The listing builds one solid part. Answer for the finished solid, in the listing's coordinates (mm). Coordinates: 2 decimals unless noted, no trailing zeros. Order: outer loops, then holes, each group sorted by start corner. A loop starts at its lowest first (then second) coordinate and runs counter-clockwise, first axis right, second up. Notation, with made-up numbers: (65, 63) -> (123, 63) arc R15 cw to (123, 88) -> close; hole circle Ø4 at (55.25, -11.5). An arc over 180 degrees is marked (long way). One line per question, with ' | ' between items.
Autodesk Inventor part; units mm, degrees
ref_plane "YZ Plane" through (0, 0, 0) normal (1, 0, 0) x (0, 1, 0)
ref_plane "XZ Plane" through (0, 0, 0) normal (0, 1, 0) x (-1, 0, 0)
ref_plane "XY Plane" through (0, 0, 0) normal (0, 0, 1) x (1, 0, 0)
sketch "Sketch1" plane through (0, 0, 0) normal (1, 0, 0) x (0, 1, 0)
  line L0 (15, 30) -> (-15, 30)
  line L1 (-15, 30) -> (-15, -30)
  line L2 (-15, -30) -> (15, -30)
  line L3 (15, -30) -> (15, 30)
  line L4 (15, 30) -> (-15, -30) construction
  line L5 (-15, 30) -> (15, -30) construction
  line L6 (15, 30) -> (18, 30)
  line L7 (18, 30) -> (18, 20)
  line L8 (18, 20) -> (15, 20)
  line L9 (15, 20) -> (15, 30)
  line L10 (15, -30) -> (18, -30)
  line L11 (18, -30) -> (18, -20)
  line L12 (18, -20) -> (15, -20)
  line L13 (15, -20) -> (15, -30)
  line L14 (15, 5) -> (18, 5)
  line L15 (18, 5) -> (18, -5)
  line L16 (18, -5) -> (15, -5)
  line L17 (15, -5) -> (15, 5)
  point P0 (0, 0)
  point P1 (18, 0)
  point P2 (0, 0)
  dimension "d0" = 30
  dimension "d1" = 60
  dimension "d2" = 3
  dimension "d3" = 10
  dimension "d4" = 3
  dimension "d5" = 10
  dimension "d6" = 3
  dimension "d7" = 10
extrude "Extrusion1" add sketch "Sketch1" along normal blind 3
sketch "Sketch2" plane through (0, 0, 0) normal (-1, 0, 0) x (0, 0, 1)
  line L0 (25, 10) -> (-25, 10)
  line L1 (-25, 10) -> (-25, -10)
  line L2 (-25, -10) -> (25, -10)
  line L3 (25, -10) -> (25, 10)
  line L4 (25, 10) -> (-25, -10) construction
  line L5 (-25, 10) -> (25, -10) construction
  line L6 (30, -15) -> (-30, -15)
  line L7 (-30, -15) -> (-30, 18)
  point P0 (0, 0)
  dimension "d10" = 5
  dimension "d11" = 5
extrude "Extrusion2" cut sketch "Sketch2" against normal blind 3
sketch "Sketch3" plane through (0, 0, 0) normal (-1, 0, 0) x (0, 0, 1)
  line L0 (-25, -10) -> (-25, 10)
  line L1 (-25, 10) -> (25, 10)
  line L2 (25, 10) -> (25, -10)
  line L3 (25, -10) -> (-25, -10)
  line L4 (-30, -15) -> (-30, 18)
  line L5 (30, -15) -> (-30, -15)
  line L6 (30, 18) -> (30, -15)
  line L7 (20, 18) -> (30, 18)
  line L8 (20, 15) -> (20, 18)
  line L9 (5, 15) -> (20, 15)
  line L10 (5, 18) -> (5, 15)
  line L11 (-5, 18) -> (5, 18)
  line L12 (-5, 15) -> (-5, 18)
  line L13 (-20, 15) -> (-5, 15)
  line L14 (-20, 18) -> (-20, 15)
  line L15 (-30, 18) -> (-20, 18)
  line L16 (25.5571, 8.6073) -> (-24.4429, -11.3927)
  line L17 (-24.4429, -11.3927) -> (-25.5571, -8.6073)
  line L18 (-25.5571, -8.6073) -> (24.4429, 11.3927)
  line L19 (24.4429, 11.3927) -> (25.5571, 8.6073)
  line L20 (25.5571, 8.6073) -> (-25.5571, -8.6073) construction
  line L21 (-24.4429, -11.3927) -> (24.4429, 11.3927) construction
  line L22 (-25.5571, 8.6073) -> (24.4429, -11.3927)
  line L23 (24.4429, -11.3927) -> (25.5571, -8.6073)
  line L24 (25.5571, -8.6073) -> (-24.4429, 11.3927)
  line L25 (-24.4429, 11.3927) -> (-25.5571, 8.6073)
  line L26 (-25.5571, 8.6073) -> (25.5571, -8.6073) construction
  line L27 (24.4429, -11.3927) -> (-24.4429, 11.3927) construction
  point P0 (0, 0)
  dimension "d14" = 3
  dimension "d15" = 3
extrude "Extrusion3" add sketch "Sketch3" against normal blind 3 contours L17 L18 L0 | L0 L18 L22 L16 L3 | L3 L16 L17 | L22 L25 L0 | L0 L1 L24 L18 L22 | L18 L24 L16 L22 | L22 L16 L24 L2 L3 | L3 L23 L22 | L25 L24 L1 | L18 L1 L2 L16 L24 | L2 L24 L23 | L18 L19 L1 | L2 L19 L16
properties part number "Back Plate"
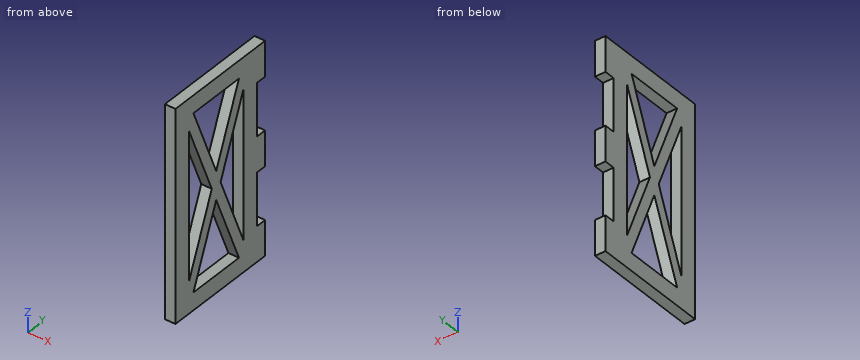
Item 1: Section A-A, the plane x = 1.85 is taken. Give the vertices of the cut face in (y, z), plus the area to 3 significant figures.
Computed values:
outline: (-15, -30) -> (18, -30) -> (18, -20) -> (15, -20) -> (15, -5) -> (18, -5) -> (18, 5) -> (15, 5) -> (15, 20) -> (18, 20) -> (18, 30) -> (-15, 30) -> close; hole (-10, -20.96) -> (-1.62, 0) -> (-10, 20.96) -> close; hole (-8.38, -25) -> (8.38, -25) -> (0, -4.04) -> close; hole (-8.38, 25) -> (0, 4.04) -> (8.38, 25) -> close; hole (1.62, 0) -> (10, -20.96) -> (10, 20.96) -> close | area: 1,190 mm^2
Item 2: This flat-tipped pin is pushed along its axis until it touches: pin 1 Ø1.5 at (x, z) = (1, 9) entering from +Y. Where does it stop, or does it pass through?
Computed values:
pin 1: stops at y = 15
Item 3: Section C-C, the plane z = 3 is taken. Give the vertices of the cut face in (x, y).
Computed values:
outline: (0, -15) -> (3, -15) -> (3, -10) -> (0, -10) -> close; (0, -2.82) -> (3, -2.82) -> (3, 2.82) -> (0, 2.82) -> close; (0, 10) -> (3, 10) -> (3, 18) -> (0, 18) -> close
Item 4: Section D-D, the plane z = 17.5 is taken. Give the vertices of the cut face in (x, y), plus the area to 3 significant figures.
Computed values:
outline: (0, -15) -> (3, -15) -> (3, -10) -> (0, -10) -> close; (0, -8.62) -> (3, -8.62) -> (3, -5.38) -> (0, -5.38) -> close; (0, 5.38) -> (3, 5.38) -> (3, 8.62) -> (0, 8.62) -> close; (0, 10) -> (3, 10) -> (3, 15) -> (0, 15) -> close | area: 49.4 mm^2
Item 5: Section B-B, the plane y = -4 is taken. Give the vertices of the cut face in (x, z), plus the area to 3 significant figures.
Computed values:
outline: (0, -30) -> (3, -30) -> (3, -25) -> (0, -25) -> close; (0, -14.04) -> (3, -14.04) -> (3, -5.96) -> (0, -5.96) -> close; (0, 5.96) -> (3, 5.96) -> (3, 14.04) -> (0, 14.04) -> close; (0, 25) -> (3, 25) -> (3, 30) -> (0, 30) -> close | area: 78.5 mm^2
Item 6: Find the intervals of material crossed by L1, parallel to Y at x = 2.3, z = -19; L2, parallel to Y at x = 1.15, z = 1; L3, parallel to Y at x = 1, z = -10.5, in increasing order.
Computed values:
L1: y = -15 to -10, -9.22 to -5.98, 5.98 to 9.22, 10 to 15 | L2: y = -15 to -10, -2.02 to 2.02, 10 to 18 | L3: y = -15 to -10, -5.82 to -2.58, 2.58 to 5.82, 10 to 15
